Here's the drawing with two shaded views (mm, measured from the low corner). I have some questions. Give positions to 0.01 mm unless a question says otherwise; leave off trailing zeros. Write each loop counter-clockwise with the first axis right and the second up, starting at its lowest first coordinate (ties: lowest second). Pieces come first, ordered by that corner, then holes.
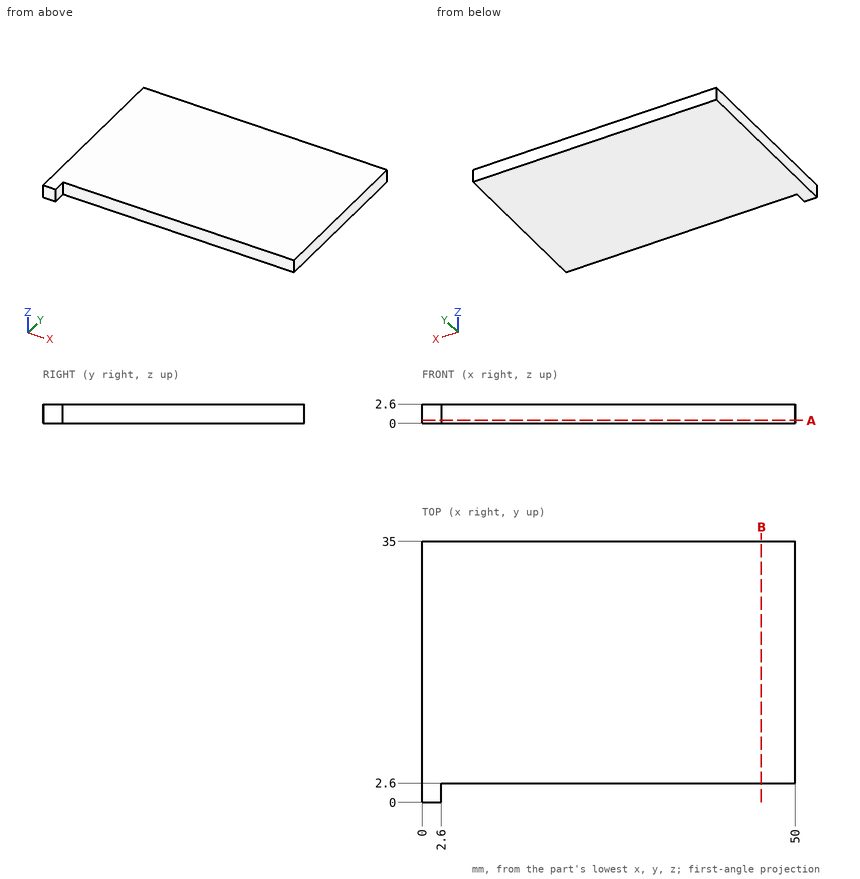
1) Suppose I cut it at B-B on x = 45.5. Write out the boundary of the cut face in (y, z).
Values follow:
outline: (2.6, 0) - (35, 0) - (35, 2.6) - (2.6, 2.6) - close
2) Suppose I cut it at A-A on z = 0.4. Write out the boundary of the cut face in (x, y), plus the area to 3 significant figures.
Values follow:
outline: (0, 0) - (2.6, 0) - (2.6, 2.6) - (50, 2.6) - (50, 35) - (0, 35) - close
area: 1,630 mm2
3) Please list where this line runs through material, in increasing order: L1, parallel to Y at x = 22.5, z = 0.3.
Values follow:
L1: y = 2.6 to 35
4) For pin 1 Ø1.3 at (y, z) = (1.5, 1.5) entering from +X; pin 2 Ø1 at (y, z) = (10.5, 1) entering from -X, each with a flat end and sliding along its axis, tell me the tip position at first contact or that it passes through.
Values follow:
pin 1: stops at x = 2.6
pin 2: stops at x = 0
